Study the drawing (mm; zero at the part's minimum x, y, z) and answer. A direction names the side the tool comes from. Round coordinates to 2 decimals unless told otherwise and drop trailing zeros. Order: outer loops, then holes, each group sorted by start corner. A loop starts at its lowest first (then second) coordinate and runs counter-clockwise, first axis right, second up. Notation, with made-up numbers: (-28.5, 38) -> (7.5, 38) arc R16 cw to (7.5, 60) -> close; hole circle Ø11 at (41, -37). An arc over 180 degrees is marked (long way). Use one line per item in the form item = value.
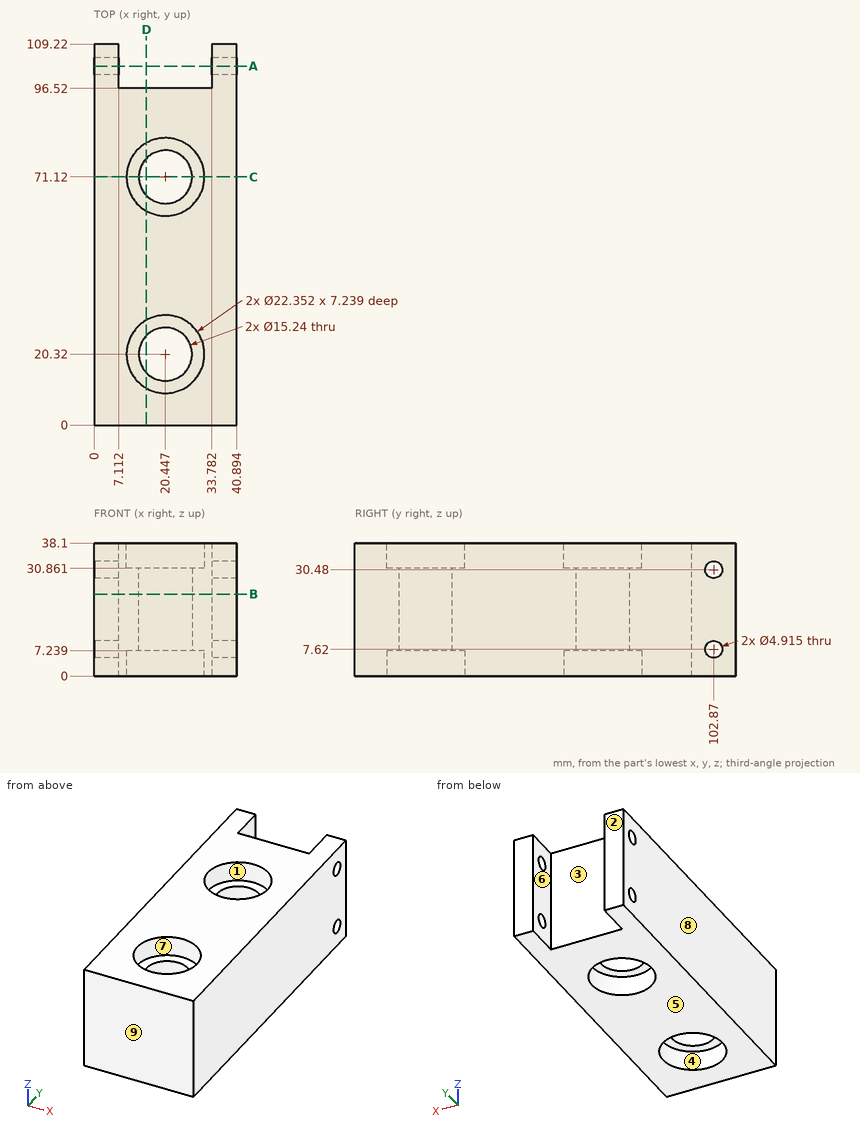
Item 1: The part is cut by section B-B, the plane z = 23.5. Give the vertices of the cut face in (x, y), and give its area (3 significant figures).
Findings:
outline = (0, 0) -> (40.89, 0) -> (40.89, 109.22) -> (33.78, 109.22) -> (33.78, 96.52) -> (7.11, 96.52) -> (7.11, 109.22) -> (0, 109.22) -> close; hole circle Ø15.24 at (20.45, 20.32); hole circle Ø15.24 at (20.45, 71.12)
area = 3,760 mm^2
Item 2: The part is cut by section C-C, the plane y = 71.12. Give the vertices of the cut face in (x, z).
Findings:
outline = (0, 0) -> (9.27, 0) -> (9.27, 7.24) -> (12.83, 7.24) -> (12.83, 30.86) -> (9.27, 30.86) -> (9.27, 38.1) -> (0, 38.1) -> close; (28.07, 7.24) -> (31.62, 7.24) -> (31.62, 0) -> (40.89, 0) -> (40.89, 38.1) -> (31.62, 38.1) -> (31.62, 30.86) -> (28.07, 30.86) -> close
Item 3: The part is cut by section A-A, the plane y = 102.87. Give the vertices of the cut face in (x, z), and give its area (3 significant figures).
Findings:
outline = (0, 0) -> (7.11, 0) -> (7.11, 5.16) -> (0, 5.16) -> close; (0, 10.08) -> (7.11, 10.08) -> (7.11, 28.02) -> (0, 28.02) -> close; (0, 32.94) -> (7.11, 32.94) -> (7.11, 38.1) -> (0, 38.1) -> close; (33.78, 0) -> (40.89, 0) -> (40.89, 5.16) -> (33.78, 5.16) -> close; (33.78, 10.08) -> (40.89, 10.08) -> (40.89, 28.02) -> (33.78, 28.02) -> close; (33.78, 32.94) -> (40.89, 32.94) -> (40.89, 38.1) -> (33.78, 38.1) -> close
area = 402 mm^2
Item 4: Determine the mould class of the marked faces 6, 7, 8 and 9 for opening direction X: released by +X, released by -X, zero draft, split by the parting line, or undercut.
Findings:
face_6 = undercut
face_7 = undercut
face_8 = released by -X
face_9 = zero draft
Item 5: The part is cut by section D-D, the plane x = 15. Give the vertices of the cut face in (y, z).
Findings:
outline = (0, 0) -> (10.56, 0) -> (10.56, 7.24) -> (14.99, 7.24) -> (14.99, 30.86) -> (10.56, 30.86) -> (10.56, 38.1) -> (0, 38.1) -> close; (25.65, 7.24) -> (30.08, 7.24) -> (30.08, 0) -> (61.36, 0) -> (61.36, 7.24) -> (65.79, 7.24) -> (65.79, 30.86) -> (61.36, 30.86) -> (61.36, 38.1) -> (30.08, 38.1) -> (30.08, 30.86) -> (25.65, 30.86) -> close; (76.45, 7.24) -> (80.88, 7.24) -> (80.88, 0) -> (96.52, 0) -> (96.52, 38.1) -> (80.88, 38.1) -> (80.88, 30.86) -> (76.45, 30.86) -> close
Item 6: For the marked faces 1, 2, 3, 4 and 5, determine the directions among +Z, -Z, +X, -X, +Y, -Y from which every point of the face is accessible in a straight line to the end or side of a thin tool.
Findings:
face_1 = +Z
face_2 = +Z, -Z, +X, -X, +Y
face_3 = +Z, -Z, +Y
face_4 = -Z
face_5 = -Z, +X, -X, +Y, -Y
Item 7: Consider line 1 along Y through (x, z) = (21, 27.5); line 2 along Y through (x, z) = (36.5, 7.62); line 3 along Y through (x, z) = (18.5, 23). Determine where each line is inside the solid, lowest interval first.
Findings:
line_1 = 0 to 12.72, 27.92 to 63.52, 78.72 to 96.52
line_2 = 0 to 100.41, 105.33 to 109.22
line_3 = 0 to 12.95, 27.69 to 63.75, 78.49 to 96.52
Item 8: Flat-ended cylindrical pins translate along their axes: P1, Ø11, axis at x = 20, y = 24.5, coming from the +Z side; P2, Ø13.5, axis at x = 19.5, z = 25, coming from the +Y side; P3, Ø6.5, axis at x = 21.5, y = 25.5, coming from the -Z side. Find the tip coordinate at first contact, or state that the pin passes through.
Findings:
P1 = 30.86
P2 = 96.52
P3 = 7.24
